Model file for the job. Use its own axes, mm. Face numbers are marked on the shaded views. Round coordinates to 2 decimals unless told otherwise and drop trailing zeros. Order: outer loops, then holes, each group sorted by start corner. A loop starts at its lowest first (then second) coordinate and runs counter-clockwise, first axis right, second up. Notation, with made-up numbers: (24, -30) -> (60, -30) arc R8 cw to (60, -20) -> close; hole circle Ø1 at (0.25, 37.25). An arc over 180 degrees is marked (long way). Put each result on its own line as item: value. Start each with the question number.
Q1. Cut at D-D, the plane y = 4. List the corners of the cut face in (x, z).
Q2. Flat gauge pins, fed straight in: P1, Ø3, axis at y = 4.5, z = -3, coming from the +X side; P2, Ø1.8, axis at x = 0, z = 7.23, coming from the +Y side; P3, Ø5, axis at x = 0, z = 0, coming from the -Y side. Where does each tip first touch, or does it go through?
Q3. Cut at C-C, the plane x = -7.23. List the corners of the cut face in (y, z), and give its area (3 significant figures).
Q4. Pull direction Z, two halves, no side cores. Call the marked faces 1, 2, 3 and 4: released by +Z, released by -Z, zero draft, split by the parting line, or undercut.
Q5. Probe L1, parallel to X at y = 4.5, z = 0; L2, parallel to X at y = 1.6, z = -3.5; L3, parallel to X at y = 1.1, z = 7.75. List the from-to ranges inside material, lowest first.
Q6. Cut at B-B, the plane z = -7. List the corners of the cut face in (x, y), and give its area (3 significant figures).
Q7. Cut at A-A, the plane y = 1.7. State how many separate pieces and enclosed holes the cut face has, and give its area (3 significant figures).
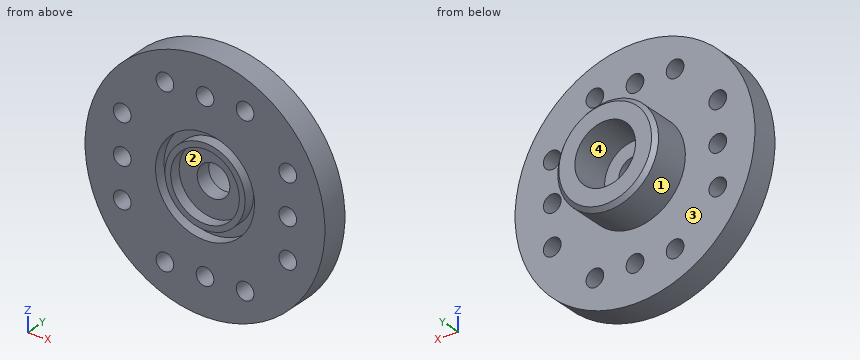
from build123d import *

# Parameters (mm, degrees)
SKETCH_2_R          = 10.475
SKETCH_2_R_2        = 4.4
SKETCH_2_R_3        = 0.771713969
EXTRUDE_1_DEPTH     = 2.35
SKETCH_3_R          = 4.4
SKETCH_3_R_2        = 2.65
EXTRUDE_2_DEPTH     = 3.5
CHAMFER_1_SIZE      = 0.35
SKETCH_4_R          = 4.4
EXTRUDE_3_DEPTH     = 2.35
SKETCH_5_R          = 3
CUT_EXTRUDE_1_DEPTH = 1
SKETCH_6_R          = 1.425
CUT_EXTRUDE_2_DEPTH = 1.35
SKETCH_7_R          = 4.325
SKETCH_7_R_2        = 3.5
CUT_EXTRUDE_3_DEPTH = 1


with BuildPart() as part:
    # Sketch 2 → Extrude 1 (new body)
    with BuildSketch(Plane(origin=(0, 0, 0), x_dir=(1, 0, 0), z_dir=(0, 1, 0))):
        with Locations(Location((0, 0, 0), (0, 0, 270))):
            Circle(SKETCH_2_R)
        with Locations(Location((0, 0, 0), (0, 0, 270))):
            Circle(SKETCH_2_R_2, mode=Mode.SUBTRACT)
        with Locations(Location((0, 7.23, 0), (0, 0, 270))):
            Circle(SKETCH_2_R_3, mode=Mode.SUBTRACT)
        with Locations(Location((-3.5, 7.23, 0), (0, 0, 270))):
            Circle(SKETCH_2_R_3, mode=Mode.SUBTRACT)
        with Locations(Location((3.5, 7.23, 0), (0, 0, 90))):
            Circle(SKETCH_2_R_3, mode=Mode.SUBTRACT)
        with Locations(Location((7.23, 3.5, 0), (0, 0, 270))):
            Circle(SKETCH_2_R_3, mode=Mode.SUBTRACT)
        with Locations(Location((7.23, 0, 0), (0, 0, 270))):
            Circle(SKETCH_2_R_3, mode=Mode.SUBTRACT)
        with Locations(Location((7.23, -3.5, 0), (0, 0, 90))):
            Circle(SKETCH_2_R_3, mode=Mode.SUBTRACT)
        with Locations(Location((3.5, -7.23, 0), (0, 0, 270))):
            Circle(SKETCH_2_R_3, mode=Mode.SUBTRACT)
        with Locations(Location((0, -7.23, 0), (0, 0, 270))):
            Circle(SKETCH_2_R_3, mode=Mode.SUBTRACT)
        with Locations(Location((-3.5, -7.23, 0), (0, 0, 90))):
            Circle(SKETCH_2_R_3, mode=Mode.SUBTRACT)
        with Locations(Location((-7.23, -3.5, 0), (0, 0, 270))):
            Circle(SKETCH_2_R_3, mode=Mode.SUBTRACT)
        with Locations(Location((-7.23, 0, 0), (0, 0, 270))):
            Circle(SKETCH_2_R_3, mode=Mode.SUBTRACT)
        with Locations(Location((-7.23, 3.5, 0), (0, 0, 90))):
            Circle(SKETCH_2_R_3, mode=Mode.SUBTRACT)
    extrude(amount=EXTRUDE_1_DEPTH)



with BuildPart() as body_2:
    # Sketch 3 → Extrude 2 (new body)
    with BuildSketch(Plane(origin=(0, 2.35, 0), x_dir=(1, 0, 0), z_dir=(0, 1, 0))):
        with Locations(Location((0, 0, 0), (0, 0, 270))):
            Circle(SKETCH_3_R)
        with Locations(Location((0, 0, 0), (0, 0, 270))):
            Circle(SKETCH_3_R_2, mode=Mode.SUBTRACT)
    extrude(amount=EXTRUDE_2_DEPTH)

    # Chamfer 1
    chamfer_1_edges = [body_2.edges().sort_by_distance(p)[0] for p in [
        (0, 5.85, -4.4),
    ]]
    chamfer(chamfer_1_edges, length=CHAMFER_1_SIZE)


with BuildPart() as part_1:
    add(part.part)

    add(body_2.part)  # Extrude 3 merges body 2
    # Sketch 4 → Extrude 3 (add)
    with BuildSketch(Plane.XZ):
        with Locations(Location((0, 0, 0), (0, 0, 270))):
            Circle(SKETCH_4_R)
    extrude(amount=-EXTRUDE_3_DEPTH)

    # Sketch 5 → Cut-Extrude 1 (cut)
    with BuildSketch(Plane.XZ):
        with Locations(Location((0, 0, 0), (0, 0, 270))):
            Circle(SKETCH_5_R)
    extrude(amount=-CUT_EXTRUDE_1_DEPTH, mode=Mode.SUBTRACT)

    # Sketch 6 → Cut-Extrude 2 (cut)
    with BuildSketch(Plane(origin=(0, 2.35, 0), x_dir=(1, 0, 0), z_dir=(0, 1, 0))):
        with Locations(Location((0, 0, 0), (0, 0, 270))):
            Circle(SKETCH_6_R)
    extrude(amount=-CUT_EXTRUDE_2_DEPTH, mode=Mode.SUBTRACT)

    # Sketch 7 → Cut-Extrude 3 (cut)
    with BuildSketch(Plane.XZ):
        with Locations(Location((0, 0, 0), (0, 0, 270))):
            Circle(SKETCH_7_R)
        with Locations(Location((0, 0, 0), (0, 0, 270))):
            Circle(SKETCH_7_R_2, mode=Mode.SUBTRACT)
    extrude(amount=-CUT_EXTRUDE_3_DEPTH, mode=Mode.SUBTRACT)


solid = part_1.part
Ans:
1. outline: circle Ø8.8 at (0, 0); hole circle Ø5.3 at (0, 0)
2. P1: stops at x = 4.14
2. P2: stops at y = 2.35
2. P3: stops at y = 1
3. outline: (0, -7.58) -> (2.35, -7.58) -> (2.35, -4.27) -> (0, -4.27) -> close; (0, -2.73) -> (2.35, -2.73) -> (2.35, -0.77) -> (0, -0.77) -> close; (0, 0.77) -> (2.35, 0.77) -> (2.35, 2.73) -> (0, 2.73) -> close; (0, 4.27) -> (2.35, 4.27) -> (2.35, 7.58) -> (0, 7.58) -> close
3. area: 24.7 mm^2
4. face 1: split by the parting line
4. face 2: undercut
4. face 3: zero draft
4. face 4: undercut
5. L1: x = -4.4 to -2.65, 2.65 to 4.4
5. L2: x = -9.87 to -8, -6.46 to 6.46, 8 to 9.87
5. L3: x = -7.05 to -4.07, -2.93 to -0.57, 0.57 to 2.93, 4.07 to 7.05
6. outline: (-7.79, 0) -> (-4.24, 0) -> (-4.24, 2.35) -> (-7.79, 2.35) -> close; (-2.76, 0) -> (-0.74, 0) -> (-0.74, 2.35) -> (-2.76, 2.35) -> close; (0.74, 0) -> (2.76, 0) -> (2.76, 2.35) -> (0.74, 2.35) -> close; (4.24, 0) -> (7.79, 0) -> (7.79, 2.35) -> (4.24, 2.35) -> close
6. area: 26.2 mm^2
7. separate pieces: 1
7. enclosed holes: 13
7. area: 316 mm^2
